Read the model definition and answer for the solid it produces. Units are mm, in the model's axes. A direction names the side the tool comes from. Coordinates: 2 decimals unless noted, no trailing zeros. Write each loop counter-clockwise with the first axis right and the second up, starting at its lowest first coordinate (ties: lowest second). Pieces come first, ordered by that corner, then holes.
(1) The mould has two halves that part along Z. Classify faces 4 (the cylindrical face through (-22.64, 5.42, 11.52)), 5 (the cylindrical face through (6.878, 5.423, -18.027)), 6 (the cylindrical face through (-17.35, 22.7, 2.36)): +Z half, -Z half, draft (parallel to the pull), parting line (faces both ways), or undercut.
(2) Section D-D on x = -6.75 is taken. Write down the section's boundary in (y, z), then the cut area to 3 significant figures.
(3) Find the intervals of material crossed by probe 1 along X at (y, z) = (10.5, 8.5); probe 2 along X at (y, z) = (18.5, -13); probe 3 along Z at (x, y) = (-13.75, 19.75), in increasing order.
(4) Section B-B on z = 1.25 is taken. Write down the section's boundary in (x, y).
(5) Section C-C on x = -20.5 is taken. Write down the section's boundary in (y, z).
(6) Given pin 1 (1.8 mm diameter, centred on y = 15.5, z = 5, fed in from +X); pin 2 (3 mm diameter, centred on x = -16, y = 14, fed in from -Z); pin 3 (1.1 mm diameter, centred on y = 14.5, z = -13, fed in from -X), each flat-ended and moving along its own axis, determine where each tip first touches the part or whether it passes through.
(7) Section A-A on y = 13 is taken. Write down the section's boundary in (x, z).
(8) Which of the six approach directions +Z, -Z, +X, -X, +Y, -Y give full straight-line access (tool end or side, diameter ignored) to faces 1 (the flat face through (-8.1, 10.5, -17.255)), 2 (the cylindrical face through (2.88, 22.7, 7.3)), 3 (the cylindrical face through (-17.35, 22.7, 7.79))?
from build123d import *

# Parameters (mm, degrees)
SKETCH1_R           = 2.5
BOSS_EXTRUDE1_DEPTH = 11
SKETCH2_R           = 3.5
CUT_EXTRUDE1_DEPTH  = 1
SKETCH3_W           = 6
SKETCH3_H           = 1
SKETCH3_W_2         = 1
SKETCH3_H_2         = 6
BOSS_EXTRUDE2_DEPTH = 13
FILLET1_R           = 1


with BuildPart() as part:
    # Sketch1 → Boss-Extrude1 (new body)
    with BuildSketch(Plane(origin=(0, 0, 0), x_dir=(1, 0, 0), z_dir=(0, 1, 0))):
        with BuildLine():
            Line((-22.081775976, 18.25540597), (6.318224024, 18.25540597))
            ThreePointArc((6.318224024, 18.25540597), (6.883909449, 18.021091395), (7.118224024, 17.45540597))
            Line((7.118224024, 17.45540597), (7.118224024, -10.94459403))
            ThreePointArc((7.118224024, -10.94459403), (6.883909449, -11.510279455), (6.318224024, -11.74459403))
            Line((6.318224024, -11.74459403), (-22.081775976, -11.74459403))
            ThreePointArc((-22.081775976, -11.74459403), (-22.647461401, -11.510279455), (-22.881775976, -10.94459403))
            Line((-22.881775976, -10.94459403), (-22.881775976, 17.45540597))
            ThreePointArc((-22.881775976, 17.45540597), (-22.647461401, 18.021091395), (-22.081775976, 18.25540597))
        make_face()
        with Locations(Location((-7.881775976, 3.25540597, 0), (0, 0, 270))):
            Circle(SKETCH1_R, mode=Mode.SUBTRACT)
    extrude(amount=BOSS_EXTRUDE1_DEPTH)

    # Sketch2 → Cut-Extrude1 (cut)
    with BuildSketch(Plane(origin=(0, 11, 0), x_dir=(1, 0, 0), z_dir=(0, 1, 0))):
        with BuildLine():
            Line((-21.381775976, 17.25540597), (5.618224024, 17.25540597))
            ThreePointArc((5.618224024, 17.25540597), (5.971777415, 17.108959361), (6.118224024, 16.75540597))
            Line((6.118224024, 16.75540597), (6.118224024, -10.24459403))
            ThreePointArc((6.118224024, -10.24459403), (5.971777415, -10.598147421), (5.618224024, -10.74459403))
            Line((5.618224024, -10.74459403), (-21.381775976, -10.74459403))
            ThreePointArc((-21.381775976, -10.74459403), (-21.735329367, -10.598147421), (-21.881775976, -10.24459403))
            Line((-21.881775976, -10.24459403), (-21.881775976, 16.75540597))
            ThreePointArc((-21.881775976, 16.75540597), (-21.735329367, 17.108959361), (-21.381775976, 17.25540597))
        make_face()
        with Locations(Location((-7.881775976, 3.25540597, 0), (0, 0, 270))):
            Circle(SKETCH2_R, mode=Mode.SUBTRACT)
    extrude(amount=-CUT_EXTRUDE1_DEPTH, mode=Mode.SUBTRACT)

    # Sketch3 → Boss-Extrude2 (add)
    with BuildSketch(Plane(origin=(0, 10, 0), x_dir=(1, 0, 0), z_dir=(0, 1, 0))):
        with Locations((-15.224035156, 12.872185426)):
            Rectangle(SKETCH3_W, SKETCH3_H)
        with Locations((0.167819541, 12.872185426)):
            Rectangle(SKETCH3_W, SKETCH3_H)
        with Locations((0.167819541, -7.304488602)):
            Rectangle(SKETCH3_W, SKETCH3_H)
        with Locations((-17.353346933, -5.074456638)):
            Rectangle(SKETCH3_W_2, SKETCH3_H_2)
    extrude(amount=BOSS_EXTRUDE2_DEPTH)

    # Fillet1
    fillet1_edges = [part.edges().sort_by_distance(p)[0] for p in [
        (-18.224035156, 23, -12.872185426),
        (-12.224035156, 23, -12.872185426),
        (-2.832180459, 23, -12.872185426),
        (3.167819541, 23, -12.872185426),
        (-2.832180459, 23, 7.304488602),
        (3.167819541, 23, 7.304488602),
        (-17.353346933, 23, 8.074456638),
        (-17.353346933, 23, 2.074456638),
    ]]
    fillet(fillet1_edges, radius=FILLET1_R)


solid = part.part
Response:
1. face 4: +Z half
1. face 5: -Z half
1. face 6: undercut
2. outline: (0, -18.26) - (11, -18.26) - (11, -17.26) - (10, -17.26) - (10, -6.57) - (11, -6.57) - (11, -5.48) - (0, -5.48) - close; (0, -1.03) - (11, -1.03) - (11, 0.06) - (10, 0.06) - (10, 10.74) - (11, 10.74) - (11, 11.74) - (0, 11.74) - close
2. area: 260 mm2
3. probe 1: x = -22.88 to -21.88, 6.12 to 7.12
3. probe 2: x = -18.22 to -12.22, -2.83 to 3.17
3. probe 3: z = -13.37 to -12.37
4. outline: (-22.88, 0) - (7.12, 0) - (7.12, 11) - (6.12, 11) - (6.12, 10) - (-21.88, 10) - (-21.88, 11) - (-22.88, 11) - close
5. outline: (0, -18.26) - (11, -18.26) - (11, -17.26) - (10, -17.26) - (10, 10.74) - (11, 10.74) - (11, 11.74) - (0, 11.74) - close
6. pin 1: stops at x = -16.85
6. pin 2: stops at z = -13.37
6. pin 3: stops at x = -18.22
7. outline: (-18.22, -13.37) - (-12.22, -13.37) - (-12.22, -12.37) - (-18.22, -12.37) - close; (-17.85, 2.07) - (-16.85, 2.07) - (-16.85, 8.07) - (-17.85, 8.07) - close; (-2.83, -13.37) - (3.17, -13.37) - (3.17, -12.37) - (-2.83, -12.37) - close; (-2.83, 6.8) - (3.17, 6.8) - (3.17, 7.8) - (-2.83, 7.8) - close
8. face 1: +Y
8. face 2: +Z, -Z, +X, +Y
8. face 3: +Z, -X, +Y
